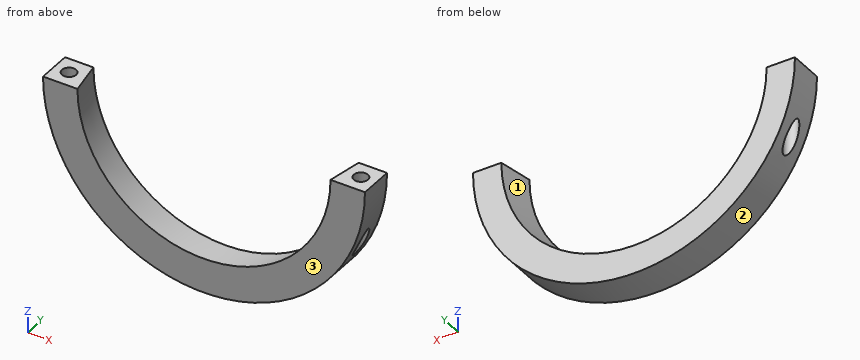
```python
from build123d import *

# Parameters (mm, degrees)
CUT_EXTRUDE3_DEPTH      = 54.524985754
CUT_EXTRUDE3_DEPTH_BACK = 54.524985754
SKETCH5_W               = 145.272182815
SKETCH5_H               = 50.443132161
M4X0_7_TAPPED_HOLE2_D   = 3.3


with BuildPart() as part:
    # Sketch3 → Revolve1 (revolve)
    with BuildSketch(Plane.XY, mode=Mode.PRIVATE) as revolve1_sk:
        Polygon((-30.810615846, 8.21), (-37.4, 8.21), (-37.4, 0.21), (-29.4, 0.21), align=None)
    revolve(revolve1_sk.sketch.rotate(Axis((0, 0, 0), (0, 1, 0)), 270), axis=Axis((0, 0, 0), (0, 1, 0)))

    # Sketch5 → Cut-Extrude3 (cut, two sides: drawn at the far end of the back side and taken through both)
    with BuildSketch(Plane(origin=(0, 0, 0), x_dir=(1, 0, 0), z_dir=(0, 1, 0)).offset(-CUT_EXTRUDE3_DEPTH_BACK)):
        with Locations((35.236091407, -25.221566081)):
            Rectangle(SKETCH5_W, SKETCH5_H)
    extrude(amount=CUT_EXTRUDE3_DEPTH + CUT_EXTRUDE3_DEPTH_BACK, mode=Mode.SUBTRACT)

    # M4x0.7 Tapped Hole2 (through all)
    with Locations(Plane.XY):
        with Locations((-33.9, 4.21), (33.9, 4.21)):
            Hole(M4X0_7_TAPPED_HOLE2_D / 2)


solid = part.part
```
Could you check a few things on this model? Use its own coordinates, in mm. Face numbers are marked on the shaded views. Give positions to 0.01 mm unless a question says otherwise; leave off trailing zeros. Write each loop counter-clockwise with the first axis right and the second up, starting at its lowest first coordinate (ties: lowest second). Pieces come first, ordered by that corner, then holes. Notation, with made-up numbers: (44, -29.5) - (84, -29.5) arc R12 ccw to (84, -18.5) - close; hole circle Ø5 at (63, -1). An arc over 180 degrees is marked (long way). One line per item, written item: value. Start each with the question number.
Item 1: Imagine slicing it at C-C, the plane z = -9.5. Give the number of separate pieces and of enclosed holes in the cut face, and give its area (3 significant figures).
Item 2: Imagine slicing it at D-D, the plane z = -33. List the corners of the cut face in (x, y) for me.
Item 3: I'm going to push flat-ended pins straight in: pin 1 (4 mm diameter, centred on y = 5.5, z = -26, fed in from -X); pin 2 (1 mm diameter, centred on y = 2, z = -6, fed in from -X); pin 3 (4 mm diameter, centred on x = 33.9, y = 4.21, fed in from -Z). Where does each tip first touch, or does it pass through?
Item 4: Imagine slicing it at A-A, the plane y = 3.5. List the corners of the cut face in (x, z) for me.
Item 5: If we mould it in two halves opening along X, with no side actions, what happens to the marked faces 1, 2 and 3? For each: +X half, -X half, draft (parallel to the pull), parting line (faces both ways), or undercut.
Item 6: Imagine slicing it at B-B, the plane x = -33.9. List the corners of the cut face in (y, z) for me, and give its area (3 significant figures).
Item 7: Please list where these lines run through material, in increasing order: line 1 (Y direction, x = 33.9, z = -6.25); line 2 (X direction, y = 4.21, z = -5); line 3 (Y direction, x = -32.5, z = -17). Write a range as from..to.
Geometry says:
1. separate pieces: 2
1. enclosed holes: 2
1. area: 105 mm^2
2. outline: (-17.6, 0.21) - (17.6, 0.21) - (17.6, 8.21) - (-17.6, 8.21) - close
3. pin 1: x = -28.68
3. pin 2: x = -36.99
3. pin 3: z = -19.52
4. outline: (-37.4, 0) arc R37.4 ccw to (-35.39, -12.1) - (-35.39, 0) - close; (-32.41, -18.66) arc R37.4 ccw to (32.41, -18.66) - (32.41, 0) - (29.98, 0) arc R29.98 cw to (-29.98, 0) - (-32.41, 0) - close; (35.39, -12.1) arc R37.4 ccw to (37.4, 0) - (35.39, 0) - close
5. face 1: undercut
5. face 2: parting line
5. face 3: draft
6. outline: (0.21, -15.8) - (2.56, -15.8) - (2.56, 0) - (0.21, 0) - close; (5.86, -15.8) - (8.21, -15.8) - (8.21, 0) - (5.86, 0) - close
6. area: 74.2 mm^2
7. line 1: 0.21..2.56, 5.86..8.21
7. line 2: -37.06..-35.55, -32.25..-29.69, 29.69..32.25, 35.55..37.06
7. line 3: 0.21..3.34, 5.08..8.21
